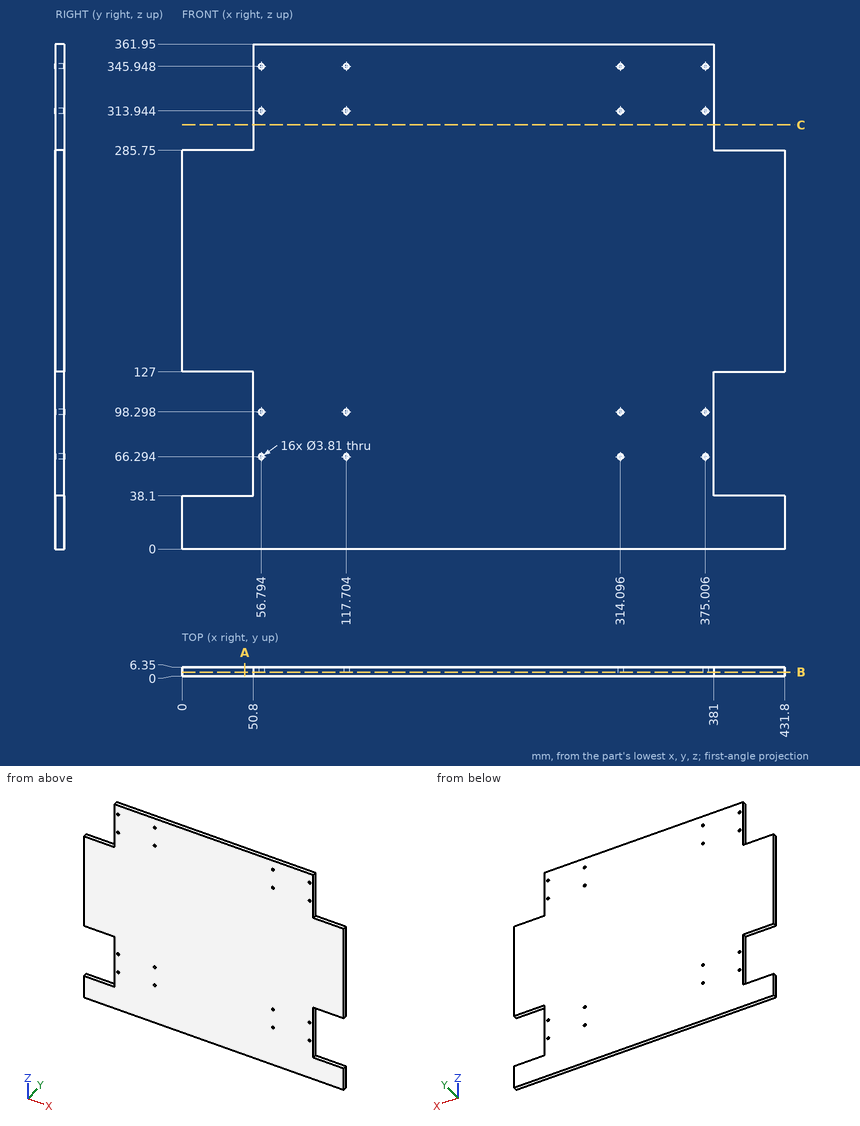
Job drawing, mm, ordinate dimensions from the low corner. One solid piece. Round coordinates to 2 decimals unless told otherwise and drop trailing zeros. Order: outer loops, then holes, each group sorted by start corner. A loop starts at its lowest first (then second) coordinate and runs counter-clockwise, first axis right, second up. Notation, with made-up numbers: (-38, -25) - (11, -25) arc R27 ccw to (11, -2) - close; hole circle Ø3 at (-33.75, 21.5). An arc over 180 degrees is marked (long way). Use CSV: the item, a comma, the result in double quotes. Start each with the question number.
1) Pin check, flat tip, straight feed: pin 1 Ø1.9 at (y, z) = (4.5, 312.5) entering from -X. Stop position of the tip, or through.
2) Saw through at B-B (y = 2.75). Count the separate pieces of the cut face and the enclosed holes in it, and give its area (3 significant figures).
3) Saw through at C-C (z = 304). List the corners of the cut face in (x, y), and give its area (3 significant figures).
4) Wall check: L1, parallel to X at y = 4.5, z = 97; L2, parallel to Z at x = 47, y = 3.75; L3, parallel to X at y = 1, z = 59.5. Give the ranges that are in metal, low to high. Write a range as [from, to].
5) Saw through at A-A (x = 45). List the corners of the cut face in (y, z), and give its area (3 significant figures).
Values follow:
1,pin 1,"stops at x = 50.8"
2,separate pieces,"1"
2,enclosed holes,"16"
2,area,"139,000 mm2"
3,outline,"(50.8, 0) - (381, 0) - (381, 6.35) - (50.8, 6.35) - close"
3,area,"2,100 mm2"
4,L1,"x = [50.8, 55.4], [58.19, 116.31], [119.1, 312.7], [315.49, 373.61], [376.4, 381]"
4,L2,"z = [0, 38.1], [127, 285.75]"
4,L3,"x = [50.8, 381]"
5,outline,"(0, 0) - (6.35, 0) - (6.35, 38.1) - (0, 38.1) - close; (0, 127) - (6.35, 127) - (6.35, 285.75) - (0, 285.75) - close"
5,area,"1,250 mm2"
